Here's how the part is built. I have some questions about the finished solid (model axes, mm). Round coordinates to 2 decimals unless told otherwise and drop trailing zeros. Loops run counter-clockwise (first coordinate to the right, second up) from the corner with the lowest first, then second, coordinate; pieces in that order, holes last. Notation, with made-up numbers: (-27, -9.5) - (-14, -9.5) arc R24 ccw to (-14, 14.5) - close; hole circle Ø2 at (63.25, 66.25). An arc over 180 degrees is marked (long way). Return JSON: item names as keys, results as strings. Group by question number.
```python
from build123d import *

# Parameters (mm, degrees)
F2_SIZE = 1
F3_SIZE = 0.5


with BuildPart() as f1:
    # F0 (on Front) → F1 (revolve)
    with BuildSketch(Plane.XZ):
        Polygon((4, 4), (4, 0), (5, 0), (5, 11), (2.5, 11), (2.5, 6), (0, 6), (0, 4), align=None)
    revolve(axis=Axis((0, 0, 2), (0, 0, 1)))

    # F2
    f2_edges = [f1.edges().sort_by_distance(p)[0] for p in [
        (-2.5, 0, 11),
    ]]
    chamfer(f2_edges, length=F2_SIZE)

    # F3
    f3_edges = [f1.edges().sort_by_distance(p)[0] for p in [
        (-4, 0, 0),
    ]]
    chamfer(f3_edges, length=F3_SIZE)


solid = f1.part
```
Q1. Will these pins go through, and if not, where does the flat tip stop? pin 1 Ø5 at (y, z) = (1, 9.5) entering from +X; pin 2 Ø2.5 at (x, y) = (0.5, -1) entering from -Z; pin 3 Ø1 at (x, y) = (1, 3.5) entering from -Z; pin 4 Ø1.5 at (x, y) = (1, -1) entering from +Z.
Q2. Please list where these lines run through material, in increasing order: line 1 (Y direction, x = 0, z = 6.95); line 2 (Y direction, x = 0, z = 1.95); line 3 (Z direction, x = 1.25, y = 1.75).
Q3. Imagine slicing it at A-A, the plane y = 0. List the corners of the cut face in (x, z) for me.
Q4. If we mould it in two halves opening along X, with no side actions, what happens to faces 1 (the cylindrical face through (-1.08, -4.88, 5.58)), 2 (the cylindrical face through (-0.867, -3.905, 2.226)), 3 (the flat face through (0, 0, 4)), 4 (the flat face through (2.2, -3.3, 11))? For each: +X half, -X half, draft (parallel to the pull), parting line (faces both ways), or undercut.
Q5. Imagine slicing it at C-C, the plane z = 8.5. List the corners of the cut face in (x, y) for me, and give its area (3 significant figures).
Q6. Imagine slicing it at D-D, the plane z = 5.25. List the corners of the cut face in (x, y) for me, and give its area (3 significant figures).
Output values:
{
 "1": {"pin 1": "stops at x = 5", "pin 2": "stops at z = 4", "pin 3": "stops at z = 0.36", "pin 4": "stops at z = 6"},
 "2": {"line 1": "y = -5 to -2.5, 2.5 to 5", "line 2": "y = -5 to -4, 4 to 5", "line 3": "z = 4 to 6"},
 "3": {"outline": "(-5, 0) - (-4.5, 0) - (-4, 0.5) - (-4, 4) - (4, 4) - (4, 0.5) - (4.5, 0) - (5, 0) - (5, 11) - (3.5, 11) - (2.5, 10) - (2.5, 6) - (-2.5, 6) - (-2.5, 10) - (-3.5, 11) - (-5, 11) - close"},
 "4": {"face 1": "parting line", "face 2": "undercut", "face 3": "undercut", "face 4": "draft"},
 "5": {"outline": "circle Ø10 at (0, 0); hole circle Ø5 at (0, 0)", "area": "58.9 mm^2"},
 "6": {"outline": "circle Ø10 at (0, 0)", "area": "78.5 mm^2"}
}
